Build history of the part. All positions in model axes, mm. Face numbers are marked on the shaded views. Round coordinates to 2 decimals unless told otherwise and drop trailing zeros. Write each loop counter-clockwise with the first axis right and the second up, starting at its lowest first coordinate (ties: lowest second). Pieces come first, ordered by that corner, then holes. Notation, with made-up numbers: (-35, 81.5) -> (21, 81.5) arc R22 ccw to (21, 111.5) -> close; hole circle Ø5 at (-29.5, 72.25). An arc over 180 degrees is marked (long way). Answer in a Markdown table with one row per item.
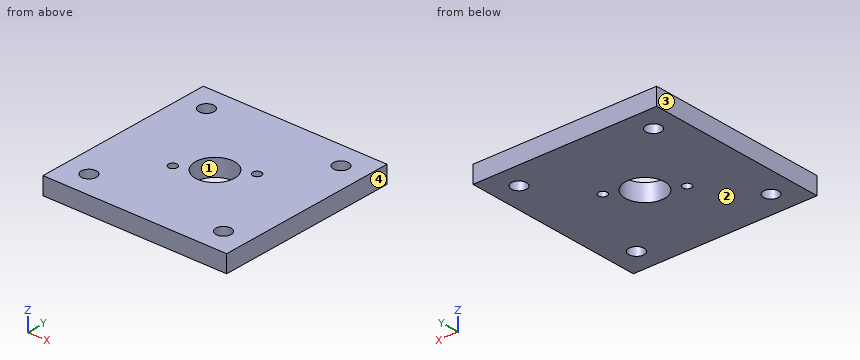
```python
from build123d import *

# Parameters (mm, degrees)
F0_W     = 42.3
F0_H     = 42.3
F1_DEPTH = 4
F2_R     = 1.75
F2_R_2   = 4.5
F2_R_3   = 1
F3_DEPTH = 25


with BuildPart() as f1:
    # F0 (on Top) → F1 (new body)
    with BuildSketch(Plane.XY):
        with Locations((-1.048587, -0.730384)):
            Rectangle(F0_W, F0_H)
    extrude(amount=F1_DEPTH)

    # F2 (on face) → F3 (cut)
    with BuildSketch(Plane.XY.offset(4)):
        with Locations((-16.548587, -16.230384)):
            Circle(F2_R)
        with Locations((14.451413, -16.230384)):
            Circle(F2_R)
        with Locations((14.451413, 14.769616)):
            Circle(F2_R)
        with Locations((-16.548587, 14.769616)):
            Circle(F2_R)
        with Locations((-1.048587, -0.730384)):
            Circle(F2_R_2)
        with Locations((-7.500477, -4.455384)):
            Circle(F2_R_3)
        with Locations((5.403302, 2.994616)):
            Circle(F2_R_3)
    extrude(amount=-F3_DEPTH, mode=Mode.SUBTRACT)


solid = f1.part
```
Q1. Saw through at D-D on x = 1.5. Write the cut outline in (y, z), plus the area to 3 significant figures.
A:
| item | result |
|---|---|
| outline | (-21.88, 0) -> (-4.44, 0) -> (-4.44, 4) -> (-21.88, 4) -> close; (2.98, 0) -> (20.42, 0) -> (20.42, 4) -> (2.98, 4) -> close |
| area | 140 mm² |
Q2. Saw through at B-B on y = 15.5. Write the cut outline in (x, z).
A:
| item | result |
|---|---|
| outline | (-22.2, 0) -> (-18.14, 0) -> (-18.14, 4) -> (-22.2, 4) -> close; (-14.96, 0) -> (12.86, 0) -> (12.86, 4) -> (-14.96, 4) -> close; (16.04, 0) -> (20.1, 0) -> (20.1, 4) -> (16.04, 4) -> close |
Q3. Drop a flat-ended pin along its axis: P1, Ø3, axis at x = -16.55, y = 14.77, coming from the -Z side. Give the stop position or say it passes through.
A:
| item | result |
|---|---|
| P1 | through |
Q4. Saw through at A-A on x = -16.5. Write the cut outline in (y, z).
A:
| item | result |
|---|---|
| outline | (-21.88, 0) -> (-17.98, 0) -> (-17.98, 4) -> (-21.88, 4) -> close; (-14.48, 0) -> (13.02, 0) -> (13.02, 4) -> (-14.48, 4) -> close; (16.52, 0) -> (20.42, 0) -> (20.42, 4) -> (16.52, 4) -> close |
Q5. Saw through at C-C on y = 0. Write the cut outline in (x, z).
A:
| item | result |
|---|---|
| outline | (-22.2, 0) -> (-5.49, 0) -> (-5.49, 4) -> (-22.2, 4) -> close; (3.39, 0) -> (20.1, 0) -> (20.1, 4) -> (3.39, 4) -> close |
Q6. Two-plate mould, pull along X, no slides. Class the marked faces 1, 2, 3 and 4: released by +X, released by -X, zero draft, split by the parting line, or undercut.
A:
| item | result |
|---|---|
| face 1 | undercut |
| face 2 | zero draft |
| face 3 | released by -X |
| face 4 | released by +X |
Q7. Wall check: line 1 (Y direction, x = 1, z = 1.5); line 2 (Y direction, x = 2, z = 3.75); line 3 (X direction, y = -15, z = 2.95). Give the ranges that are in metal, low to high. Write a range as [from, to].
A:
| item | result |
|---|---|
| line 1 | [-21.88, -4.74], [3.28, 20.42] |
| line 2 | [-21.88, -4.04], [2.58, 20.42] |
| line 3 | [-22.2, -17.79], [-15.3, 13.21], [15.7, 20.1] |
